Source: CAD feature listing. Evaluate the final solid. Frame: model axes, mm. Face numbers are marked on the shaded views. Coordinates: 2 decimals unless noted, no trailing zeros. Order: outer loops, then holes, each group sorted by start corner. A loop starts at its lowest first (then second) coordinate and runs counter-clockwise, first axis right, second up.
Autodesk Fusion 360 part; units mm, degrees
sketch "Sketch1" plane through (0, 0, 0) normal (0, 0, 1) x (1, 0, 0)
  line L0 (-12.7, 11.15) -> (12.7, 11.15)
  line L1 (12.7, 11.15) -> (12.7, -11.15)
  line L2 (12.7, -11.15) -> (-12.7, -11.15)
  line L3 (-12.7, -11.15) -> (-12.7, 11.15)
  line L4 (0, 0) -> (0, 28.3109) construction
  line L5 (0, 0) -> (22.2982, 0) construction
  circle A0 centre (11.4, 8.65) radius 0.6
  circle A1 centre (11.4, 6.65) radius 0.6
  circle A2 centre (11.4, 4.65) radius 0.6
  circle A3 centre (11.4, 2.65) radius 0.6
  circle A4 centre (11.4, 0.65) radius 0.6
  circle A5 centre (11.4, -1.35) radius 0.6
  circle A6 centre (11.4, -3.35) radius 0.6
  circle A7 centre (11.4, -5.35) radius 0.6
  circle A8 centre (11.4, -7.35) radius 0.6
  circle A9 centre (11.4, -9.35) radius 0.6
  circle A10 centre (-11.4, 0.35) radius 0.6
  circle A11 centre (-11.4, -1.65) radius 0.6
  circle A12 centre (-11.4, -3.65) radius 0.6
  circle A13 centre (-11.4, -5.65) radius 0.6
  circle A14 centre (-11.4, -7.65) radius 0.6
  circle A15 centre (-11.4, 9.85) radius 0.6
  circle A16 centre (-11.4, 7.85) radius 0.6
  circle A17 centre (-11.4, 5.85) radius 0.6
  circle A18 centre (-11.4, 3.85) radius 0.6
  dimension "d1" = 22.3
  dimension "d2" = 25.4
  dimension "d3" = 2.5
  dimension "d4" = 1.2
  dimension "d5" = 1.3
  dimension "d8" = 0
  dimension "d9" = -18
  dimension "d10" = 1.2
  dimension "d11" = 1.3
  dimension "d12" = 10.8
  dimension "d15" = 0
  dimension "d16" = -8
  dimension "d17" = 1.2
  dimension "d18" = 1.3
  dimension "d19" = 1.3
  dimension "d22" = 0
  dimension "d23" = -6
extrude "Extrude1" add sketch "Sketch1" along normal blind 1.2
sketch "Sketch2" plane through (0, 0, 1.2) normal (0, 0, 1) x (-1, 0, 0)
  circle A0 centre (11.4, 5.65) radius 0.6
  circle A1 centre (-11.4, -8.65) radius 0.6
  circle A2 centre (11.4, -9.85) radius 0.6
  circle A3 centre (11.4, 3.65) radius 0.6
  circle A4 centre (-11.4, -4.65) radius 0.6
  circle A5 centre (-11.4, -6.65) radius 0.6
  circle A6 centre (11.4, 7.65) radius 0.6
  circle A7 centre (11.4, -0.35) radius 0.6
  circle A8 centre (-11.4, 5.35) radius 0.6
  circle A9 centre (-11.4, 7.35) radius 0.6
  circle A10 centre (-11.4, -0.65) radius 0.6
  circle A11 centre (-11.4, 9.35) radius 0.6
  circle A12 centre (-11.4, -2.65) radius 0.6
  circle A13 centre (-11.4, 3.35) radius 0.6
  circle A14 centre (11.4, -7.85) radius 0.6
  circle A15 centre (11.4, -5.85) radius 0.6
  circle A16 centre (11.4, -3.85) radius 0.6
  circle A17 centre (11.4, 1.65) radius 0.6
  circle A18 centre (-11.4, 1.35) radius 0.6
  line L0 (12.7, 11.15) -> (-12.7, 11.15)
  line L1 (-12.7, 11.15) -> (-12.7, -11.15)
  line L2 (-12.7, -11.15) -> (12.7, -11.15)
  line L3 (12.7, -11.15) -> (12.7, 11.15)
  circle A19 centre (0, 0) radius 10
  dimension "d26" = 20
extrude "Extrude2" add sketch "Sketch2" along normal blind 13.6 contours A19
ref_plane "WorkPlane1" through (0, 0, 14.8) normal (0, 0, 1) x (-1, 0, 0)
sketch "Sketch3" plane through (0, 0, 14.8) normal (0, 0, 1) x (1, 0, 0)
  circle A0 centre (0, 0) radius 10.5
  dimension "d30" = 21
extrude "Extrude3" add sketch "Sketch3" along normal blind 3.4
fillet "Fillet1" radius 1 1 edges at (-9.7894, -3.797, 18.2)
sketch "Sketch4" plane through (0, 0, 1.2) normal (0, 0, 1) x (-1, 0, 0)
  circle A0 centre (0, 0) radius 10
  circle A1 centre (11.4, 5.65) radius 0.6
  circle A2 centre (-11.4, -8.65) radius 0.6
  circle A3 centre (11.4, -9.85) radius 0.6
  circle A4 centre (11.4, 3.65) radius 0.6
  circle A5 centre (-11.4, -4.65) radius 0.6
  circle A6 centre (-11.4, -6.65) radius 0.6
  circle A7 centre (11.4, 7.65) radius 0.6
  circle A8 centre (11.4, -0.35) radius 0.6
  circle A9 centre (-11.4, 5.35) radius 0.6
  circle A10 centre (-11.4, 7.35) radius 0.6
  circle A11 centre (-11.4, -0.65) radius 0.6
  circle A12 centre (-11.4, 9.35) radius 0.6
  circle A13 centre (-11.4, -2.65) radius 0.6
  circle A14 centre (-11.4, 3.35) radius 0.6
  circle A15 centre (11.4, -7.85) radius 0.6
  circle A16 centre (11.4, -5.85) radius 0.6
  circle A17 centre (11.4, -3.85) radius 0.6
  circle A18 centre (11.4, 1.65) radius 0.6
  circle A19 centre (-11.4, 1.35) radius 0.6
  line L0 (12.7, 11.15) -> (-12.7, 11.15)
  line L1 (-12.7, 11.15) -> (-12.7, -11.15)
  line L2 (-12.7, -11.15) -> (12.7, -11.15)
  line L3 (12.7, -11.15) -> (12.7, 11.15)
ref_plane "WorkPlane2" through (0, 0, 14.8) normal (0, 0, -1) x (-1, 0, 0)
sketch "Sketch5" plane through (0, 0, 14.8) normal (0, 0, -1) x (-1, 0, 0)
ref_plane "WorkPlane3" through (0, 0, 14.8) normal (0, 0, -1) x (-1, 0, 0)
sketch "Sketch6" plane through (0, 0, 14.8) normal (0, 0, -1) x (-1, 0, 0)
  line L0 (-9.3153, -2.737) -> (-7.4198, -6.2594)
  line L1 (-7.4198, -6.2594) -> (-8.3004, -6.7333)
  line L2 (-8.3004, -6.7333) -> (-10.1959, -3.2109)
  line L3 (-10.1959, -3.2109) -> (-9.3153, -2.737)
  circle A0 centre (0, 0) radius 9.5
  dimension "d37" = 4
  dimension "d38" = 1
  dimension "d39" = 4
extrude "Extrude4" add sketch "Sketch6" along normal blind 13.6 contours L0 L1 L2 L3
sketch "Sketch7" plane through (0, 0, 0) normal (0, 0, -1) x (1, 0, 0)
  circle A0 centre (-11.4, 5.65) radius 0.6
  circle A1 centre (11.4, -8.65) radius 0.6
  circle A2 centre (-11.4, -9.85) radius 0.6
  circle A3 centre (-11.4, 3.65) radius 0.6
  circle A4 centre (11.4, -4.65) radius 0.6
  circle A5 centre (11.4, -6.65) radius 0.6
  circle A6 centre (-11.4, 7.65) radius 0.6
  circle A7 centre (-11.4, -0.35) radius 0.6
  circle A8 centre (11.4, 5.35) radius 0.6
  circle A9 centre (11.4, 7.35) radius 0.6
  circle A10 centre (11.4, -0.65) radius 0.6
  circle A11 centre (11.4, 9.35) radius 0.6
  circle A12 centre (11.4, -2.65) radius 0.6
  circle A13 centre (11.4, 3.35) radius 0.6
  circle A14 centre (-11.4, -7.85) radius 0.6
  circle A15 centre (-11.4, -5.85) radius 0.6
  circle A16 centre (-11.4, -3.85) radius 0.6
  circle A17 centre (-11.4, 1.65) radius 0.6
  circle A18 centre (11.4, 1.35) radius 0.6
  line L0 (12.7, 11.15) -> (-12.7, 11.15)
  line L1 (-12.7, 11.15) -> (-12.7, -11.15)
  line L2 (-12.7, -11.15) -> (12.7, -11.15)
  line L3 (12.7, -11.15) -> (12.7, 11.15)
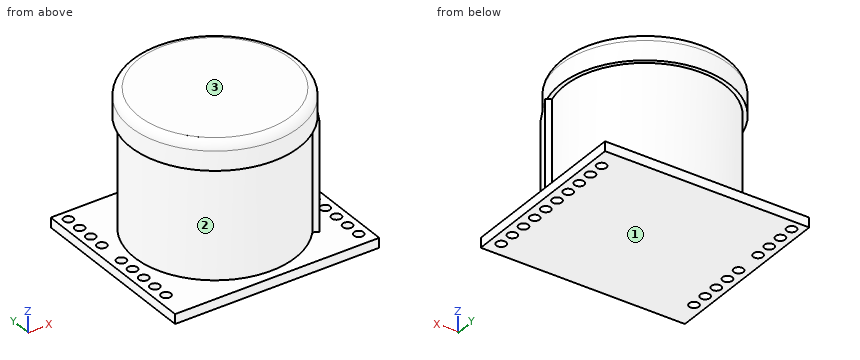
Q1. Pull-direction query (Z, two-part tool) for the marked faces 1, 2 and 3; classes: pulls with the +Z half, pulls with the -Z half, needs draft (parallel to the pull), parting line crosses it, or undercut.
Solutions:
face 1: pulls with the -Z half
face 2: undercut
face 3: pulls with the +Z half
Q2. Pin query (flat end, axial travel): P1, Ø0.8, axis at x = 10, y = -4.5, coming from the +Z side; P2, Ø1, axis at x = 8.5, z = 2, coming from the +Y side; P3, Ø10, axis at y = 5, z = 15, coming from the +X side. Return the tip coordinate at first contact, or that it passes through.
Solutions:
P1: stops at z = 1.2
P2: stops at y = 6
P3: stops at x = 10.5
Q3. Section query A-A on x = 0. Output: boundary loops of the cut face in (y, z), plus the area to 3 significant figures.
Solutions:
outline: (-11.15, 0) - (11.15, 0) - (11.15, 1.2) - (10, 1.2) - (10, 14.8) - (10.5, 14.8) - (10.5, 17.2) arc R1 ccw to (9.5, 18.2) - (-9.5, 18.2) arc R1 ccw to (-10.5, 17.2) - (-10.5, 14.8) - (-10, 14.8) - (-10, 1.2) - (-11.15, 1.2) - close
area: 370 mm2
Q4. Material intervals for line 1 along Z through (x, y) = (10.5, 7); line 2 along X through (y, z) = (-0.25, 9.5); line 3 along Y through (x, z) = (-0.25, 16.25), sorted ascending.
Solutions:
line 1: z = 0 to 1.2
line 2: x = -10 to 10
line 3: y = -10.5 to 10.5
Q5. Section query C-C on z = 2.75. Output: boundary loops of the cut face in (x, y).
Solutions:
outline: (7.68, -6.4) - (8.3, -6.73) - (10.2, -3.21) - (9.58, -2.88) arc R10 ccw (long way) to start
Q6. Section query B-B on x = -11.4. Give the number of separate pieces and of enclosed holes in the cut face, plus the area to 3 significant figures.
Solutions:
separate pieces: 10
enclosed holes: 0
area: 13.8 mm2
